```python
from build123d import *

# Parameters (mm, degrees)
SKETCH2_W                                       = 57.5
SKETCH2_H                                       = 57.5
BOSS_EXTRUDE1_DEPTH                             = 4
CUT_EXTRUDE4_DEPTH                              = 2.4
M3_CLEARANCE_HOLE1_D                            = 3.4
CSK_FOR_M3_FLAT_HEAD_MACHINE_SCREW1_D           = 3.4
CSK_FOR_M3_FLAT_HEAD_MACHINE_SCREW1_CSINK_D     = 6.3
CSK_FOR_M3_FLAT_HEAD_MACHINE_SCREW1_CSINK_ANGLE = 90
SKETCH11_W                                      = 17.5
SKETCH11_H                                      = 20
CUT_EXTRUDE3_DEPTH                              = 82.415600471
FILLET1_R                                       = 2
CUT_EXTRUDE6_DEPTH                              = 2.4
M3_CLEARANCE_HOLE2_D                            = 3.4
CHAMFER1_SIZE                                   = 5


with BuildPart() as part:
    # Sketch2 → Boss-Extrude1 (new body)
    with BuildSketch(Plane.XY):
        with Locations((28.75, 28.75)):
            Rectangle(SKETCH2_W, SKETCH2_H)
    extrude(amount=BOSS_EXTRUDE1_DEPTH)

    # Sketch12 → Cut-Extrude4 (cut)
    with BuildSketch(Plane.XY):
        Polygon((45, 41.766838493), (47.8, 43.383419246), (47.8, 46.616580754), (45, 48.233161507), (42.2, 46.616580754), (42.2, 43.383419246), align=None)
    extrude(amount=CUT_EXTRUDE4_DEPTH, mode=Mode.SUBTRACT)

    # M3 Clearance Hole1 (through all)
    with Locations(Plane.XY.offset(4)):
        with Locations((45, 45), (-45, 45), (-45, -45), (45, -45)):
            Hole(M3_CLEARANCE_HOLE1_D / 2)

    # CSK for M3 Flat Head Machine Screw1 (through all)
    with Locations(Plane.XY.offset(4)):
        with Locations((0, 50), (0, 0), (48, 0)):
            CounterSinkHole(CSK_FOR_M3_FLAT_HEAD_MACHINE_SCREW1_D / 2, CSK_FOR_M3_FLAT_HEAD_MACHINE_SCREW1_CSINK_D / 2, counter_sink_angle=CSK_FOR_M3_FLAT_HEAD_MACHINE_SCREW1_CSINK_ANGLE)

    # Sketch11 → Cut-Extrude3 (cut, through all)
    with BuildSketch(Plane.XY):
        with Locations((20.75, 28)):
            Rectangle(SKETCH11_W, SKETCH11_H)
    extrude(amount=CUT_EXTRUDE3_DEPTH, mode=Mode.SUBTRACT)

    # Fillet1
    fillet1_edges = [part.edges().sort_by_distance(p)[0] for p in [
        (29.5, 38, 2),
        (12, 38, 2),
        (12, 18, 2),
        (29.5, 18, 2),
    ]]
    fillet(fillet1_edges, radius=FILLET1_R)

    # Sketch15 → Cut-Extrude6 (cut)
    with BuildSketch(Plane.XY):
        Polygon((54.286190427, 49.713809573), (55.122994201, 52.836803774), (52.836803774, 55.122994201), (49.713809573, 54.286190427), (48.877005799, 51.163196226), (51.163196226, 48.877005799), align=None)
    extrude(amount=CUT_EXTRUDE6_DEPTH, mode=Mode.SUBTRACT)

    # M3 Clearance Hole2 (through all)
    with Locations(Plane(origin=(0, 0, 0), x_dir=(-1, 0, 0), z_dir=(0, 0, -1))):
        with Locations((-52, 52)):
            Hole(M3_CLEARANCE_HOLE2_D / 2)

    # Chamfer1
    chamfer1_edges = [part.edges().sort_by_distance(p)[0] for p in [
        (57.5, 57.5, 2),
    ]]
    chamfer(chamfer1_edges, length=CHAMFER1_SIZE)

    # Mirror1: part across plane


with BuildPart() as part_1:
    add(part.part)
    add(part.part.mirror(Plane(origin=(0, 0, 0), x_dir=(0, 0, 1), z_dir=(0, -1, 0))))

    # Mirror2: part across plane


with BuildPart() as part_2:
    add(part_1.part)
    add(part_1.part.mirror(Plane(origin=(0, 0, 0), x_dir=(0, 0, 1), z_dir=(1, 0, 0))))


solid = part_2.part
```
The listing builds one solid part. Answer for the finished solid, in the listing's coordinates (mm). A direction names the side the tool comes from. Give positions to 0.01 mm unless a question says otherwise; leave off trailing zeros. Loops run counter-clockwise (first coordinate to the right, second up) from the corner with the lowest first, then second, coordinate; pieces in that order, holes last. Notation, with made-up numbers: (6.5, 89.25) - (28.5, 89.25) arc R36 ccw to (28.5, 127.25) - close; hole circle Ø5 at (-30.5, -5.75). An arc over 180 degrees is marked (long way). Return JSON: item names as keys, results as strings. Group by question number.
1. Determine the mould class of faces 3 (the flat face through (-21, 18, 2)), 4 (the flat face through (55, -55, 2)), 5 (the flat face through (-55, -55, 2)) for opening direction X: pulls with the +X half, pulls with the -X half, needs draft (parallel to the pull), parting line crosses it, or undercut.
2. Given pin 1 Ø4 at (x, y) = (-45, 45) entering from -Z; pin 2 Ø3 at (x, y) = (-52, 52) entering from +Z; pin 3 Ø4 at (x, y) = (45, -45) entering from +Z, each flat-ended and moving along its own axis, determine where each tip first touches the part or whether it passes through.
3. Which of the six approach directions +Z, -Z, +X, -X, +Y, -Y give full straight-line access (tool end or side, diameter ignored) to faces 1 (the flat face through (-29.5, 28, 2)), 2 (the flat face through (-53.34, 50.66, 2.4))?
4. Find section A-A (y = 0). Write down the section's boundary in (x, z).
5. Straight lines are drawn through the part: line 1 (X direction, y = -45, z = 3.4); line 2 (Y direction, x = 52, z = 2.9). For each, find the intervals that lie inside material, in ascending order. Write a range as [from, to].
6. Find section B-B (z = 1.55). State how many separate pieces and enclosed holes the cut face has, then the cut area to 3 significant figures.
Verdict:
{
 "1": {"face 3": "undercut", "face 4": "pulls with the +X half", "face 5": "pulls with the -X half"},
 "2": {"pin 1": "stops at z = 2.4", "pin 2": "passes through", "pin 3": "stops at z = 4"},
 "3": {"face 1": "+Z, -Z", "face 2": "-Z"},
 "4": {"outline": "(-57.5, 0) - (-49.7, 0) - (-49.7, 2.55) - (-51.15, 4) - (-57.5, 4) - close; (-46.3, 0) - (-1.7, 0) - (-1.7, 2.55) - (-3.15, 4) - (-44.85, 4) - (-46.3, 2.55) - close; (1.7, 0) - (46.3, 0) - (46.3, 2.55) - (44.85, 4) - (3.15, 4) - (1.7, 2.55) - close; (49.7, 0) - (57.5, 0) - (57.5, 4) - (51.15, 4) - (49.7, 2.55) - close"},
 "5": {"line 1": "x = [-57.5, -46.7], [-43.3, 43.3], [46.7, 57.5]", "line 2": "y = [-57.5, -53.7], [-50.3, 50.3], [53.7, 57.5]"},
 "6": {"separate pieces": "1", "enclosed holes": "17", "area": "11,500 mm^2"}
}
